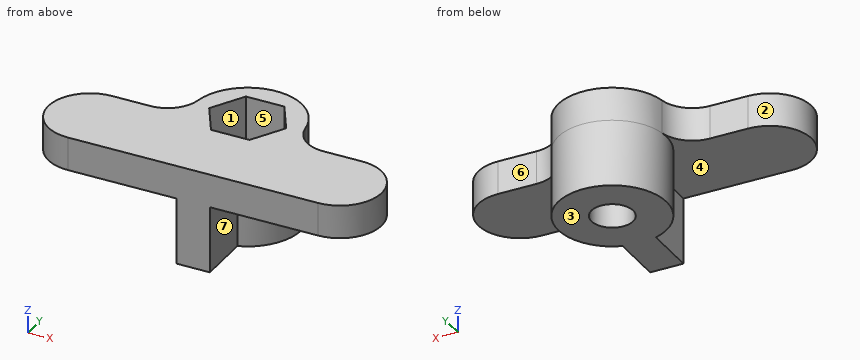
from build123d import *

# Parameters (mm, degrees)
SKETCH1_R           = 1.25
BOSS_EXTRUDE1_DEPTH = 2
BOSS_EXTRUDE2_DEPTH = 4
FILLET1_R           = 2
SKETCH3_R           = 1.25
BOSS_EXTRUDE3_DEPTH = 4
BOSS_EXTRUDE4_DEPTH = 2
CUT_EXTRUDE1_DEPTH  = 4


with BuildPart() as part:
    # Sketch1 → Boss-Extrude1 (new body)
    with BuildSketch(Plane.XY):
        with BuildLine():
            Line((-7.5, -1.25), (-3, -1.25))
            ThreePointArc((-3, -1.25), (0, 3.25), (3, -1.25))
            Line((3, -1.25), (7.5, -1.25))
            ThreePointArc((7.5, -1.25), (10, -3.75), (7.5, -6.25))
            Line((7.5, -6.25), (-7.5, -6.25))
            ThreePointArc((-7.5, -6.25), (-10, -3.75), (-7.5, -1.25))
        make_face()
        Circle(SKETCH1_R, mode=Mode.SUBTRACT)
    extrude(amount=BOSS_EXTRUDE1_DEPTH)

    # Sketch2 → Boss-Extrude2 (add)
    with BuildSketch(Plane.XY.offset(2)):
        with BuildLine():
            Line((-8, -6.199489743), (-8, -1.300510257))
            ThreePointArc((-8, -1.300510257), (-10, -3.75), (-8, -6.199489743))
        make_face()
        with BuildLine():
            ThreePointArc((3, -1.703672504), (0, -3.45), (-3, -1.703672504))
            Line((-3, -1.703672504), (-3, -6.25))
            Line((-3, -6.25), (3, -6.25))
            Line((3, -6.25), (3, -1.703672504))
        make_face()
        with BuildLine():
            ThreePointArc((8, -6.199489743), (10, -3.75), (8, -1.300510257))
            Line((8, -1.300510257), (8, -6.199489743))
        make_face()
    extrude(amount=BOSS_EXTRUDE2_DEPTH)

    # Fillet1
    fillet1_edges = [part.edges().sort_by_distance(p)[0] for p in [
        (3, -1.25, 1),
        (-3, -1.25, 1),
    ]]
    fillet(fillet1_edges, radius=FILLET1_R)


with BuildPart() as body_2:
    # Sketch3 → Boss-Extrude3 (new body)
    with BuildSketch(Plane.XY.offset(2)):
        with BuildLine():
            Line((-1, -3.092329219), (-1, -6.25))
            Line((-1, -6.25), (1, -6.25))
            Line((1, -6.25), (1, -3.092329219))
            ThreePointArc((1, -3.092329219), (0, 3.25), (-1, -3.092329219))
        make_face()
        Circle(SKETCH3_R, mode=Mode.SUBTRACT)
    extrude(amount=BOSS_EXTRUDE3_DEPTH)

    # Sketch4 → Boss-Extrude4 (add)
    with BuildSketch(Plane.XY.offset(6)):
        with BuildLine():
            Line((7.5, -1.25), (5.196152423, -1.25))
            ThreePointArc((5.196152423, -1.25), (3.886845081, -0.761857892), (3.216665785, 0.464285714))
            ThreePointArc((3.216665785, 0.464285714), (0, 3.25), (-3.216665785, 0.464285714))
            ThreePointArc((-3.216665785, 0.464285714), (-3.886845081, -0.761857892), (-5.196152423, -1.25))
            Line((-5.196152423, -1.25), (-7.5, -1.25))
            ThreePointArc((-7.5, -1.25), (-10, -3.75), (-7.5, -6.25))
            Line((-7.5, -6.25), (7.5, -6.25))
            ThreePointArc((7.5, -6.25), (10, -3.75), (7.5, -1.25))
        make_face()
    extrude(amount=BOSS_EXTRUDE4_DEPTH)

    # Sketch5 → Cut-Extrude1 (cut)
    with BuildSketch(Plane.XY.offset(8)):
        Polygon((1.154700538, 2), (-1.154700538, 2), (-2.309401077, 0), (-1.154700538, -2), (1.154700538, -2), (2.309401077, 0), align=None)
    extrude(amount=-CUT_EXTRUDE1_DEPTH, mode=Mode.SUBTRACT)


solid = body_2.part
The model under review builds one solid part; all positions refer to its coordinate system, in mm. Face numbers are marked on the shaded views. A direction names the side the tool comes from. Coordinates: 2 decimals unless noted, no trailing zeros. Loops run counter-clockwise (first coordinate to the right, second up) from the corner with the lowest first, then second, coordinate; pieces in that order, holes last. Notation, with made-up numbers: (89, 69) -> (130, 69) arc R16 cw to (130, 95) -> close; hole circle Ø1 at (7.25, 1.25). An arc over 180 degrees is marked (long way). Use a Markdown table: item, result. Add a question column.
1. Add section C-C on z = 3.5. Write out the cut boundary in (x, y), plus the area to 3 significant figures.
2. Machinability: for the marked faces 4, 5, 6 and 7, which of the approach directions +Z, -Z, +X, -X, +Y, -Y give a long, thin tool a straight path to every point of the face, cutting with its end or side? Answer none if there is none.
3. Add section B-B on y = -0.75. Write out the cut boundary in (x, z), plus the area to 3 significant figures.
4. Add section A-A on x = 0. Write out the cut boundary in (y, z).
5. Clearance check with flat-ended pins moving along their axes: pin 1 Ø3 at (x, y) = (-0.5, 0) entering from +Z; pin 2 Ø1.5 at (y, z) = (1.5, 7) entering from -X; pin 3 Ø5.5 at (x, y) = (5.5, -4.5) entering from -Z; pin 4 Ø1 at (x, y) = (-4.5, -0.5) entering from -Z. State where each tip first meets the part, or that it passes through.
6. To check wall thickness, follow line 1 (X direction, y = 0, z = 3.35); line 2 (Y direction, x = 0, z = 2.6); line 3 (Z direction, x = -1.5, y = -4.5). State the ranges of each line that lie inside material, in increasing order.
7. Draft analysis for pull direction X (two halves, no side actions). For the marked faces 1, 2 and 3, state which applies: pulls with the +X half, pulls with the -X half, needs draft (parallel to the pull), parting line crosses it, or undercut.
8. Add section D-D on y = 0.75. Write out the cut boundary in (x, z), plus the area to 3 significant figures.
Returned:
| question | item | result |
|---|---|---|
| 1 | outline | (-1, -6.25) -> (1, -6.25) -> (1, -3.09) arc R3.25 ccw (long way) to (-1, -3.09) -> close; hole circle Ø2.5 at (0, 0) |
| 1 | area | 34.4 mm² |
| 2 | face 4 | -Z, -X, -Y |
| 2 | face 5 | +Z |
| 2 | face 6 | +Z, -Z, +X, +Y |
| 2 | face 7 | -Z, +X, -Y |
| 3 | outline | (-3.87, 6) -> (-3.16, 6) -> (-3.16, 2) -> (-1, 2) -> (-1, 4) -> (-1.88, 4) -> (-1.88, 8) -> (-3.87, 8) -> close; (1, 2) -> (3.16, 2) -> (3.16, 6) -> (3.87, 6) -> (3.87, 8) -> (1.88, 8) -> (1.88, 4) -> (1, 4) -> close |
| 3 | area | 21.8 mm² |
| 4 | outline | (-6.25, 2) -> (-1.25, 2) -> (-1.25, 4) -> (-2, 4) -> (-2, 8) -> (-6.25, 8) -> close; (1.25, 2) -> (3.25, 2) -> (3.25, 8) -> (2, 8) -> (2, 4) -> (1.25, 4) -> close |
| 5 | pin 1 | stops at z = 4 |
| 5 | pin 2 | stops at x = -3.16 |
| 5 | pin 3 | stops at z = 6 |
| 5 | pin 4 | passes through |
| 6 | line 1 | x = -3.25 to -1.25, 1.25 to 3.25 |
| 6 | line 2 | y = -6.25 to -1.25, 1.25 to 3.25 |
| 6 | line 3 | z = 6 to 8 |
| 7 | face 1 | undercut |
| 7 | face 2 | pulls with the -X half |
| 7 | face 3 | needs draft |
| 8 | outline | (-3.16, 2) -> (-1, 2) -> (-1, 4) -> (-1.88, 4) -> (-1.88, 8) -> (-3.16, 8) -> close; (1, 2) -> (3.16, 2) -> (3.16, 8) -> (1.88, 8) -> (1.88, 4) -> (1, 4) -> close |
| 8 | area | 18.9 mm² |
